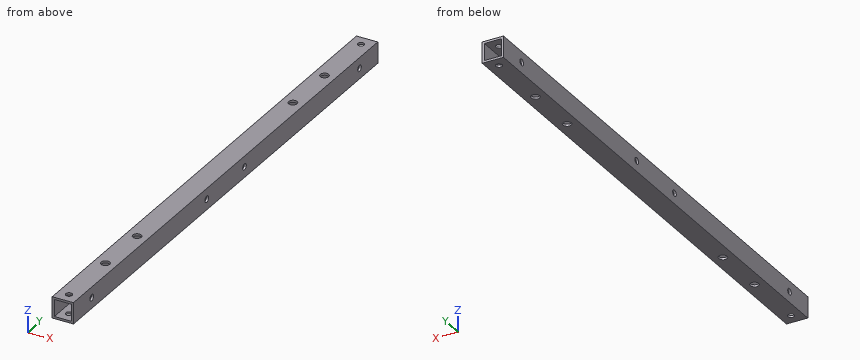
```python
from build123d import *

# Parameters (mm, degrees)
F0_W     = 10
F0_H     = 10
F0_W_2   = 8
F0_H_2   = 8
F1_DEPTH = 250
F2_R     = 1.5
F4_DEPTH = 25
F3_R     = 1.5
F3_R_2   = 2
F5_DEPTH = 25


with BuildPart() as f1:
    # F0 (on Front) → F1 (new body)
    with BuildSketch(Plane.XZ):
        Rectangle(F0_W, F0_H)
        Rectangle(F0_W_2, F0_H_2, mode=Mode.SUBTRACT)
    extrude(amount=F1_DEPTH)

    # F2 (on face) → F4 (cut)
    with BuildSketch(Plane.YZ.offset(5)):
        with Locations((-140.5, 0)):
            Circle(F2_R)
        with Locations((-235, 0)):
            Circle(F2_R)
        with Locations((-15, 0)):
            Circle(F2_R)
        with Locations((-109.5, 0)):
            Circle(F2_R)
    extrude(amount=-F4_DEPTH, mode=Mode.SUBTRACT)

    # F3 (on face) → F5 (cut)
    with BuildSketch(Plane.XY.offset(5)):
        with Locations((0, -245)):
            Circle(F3_R)
        with Locations((0, -215)):
            Circle(F3_R_2)
        with Locations((0, -189)):
            Circle(F3_R_2)
        with Locations((0, -61)):
            Circle(F3_R_2)
        with Locations((0, -35)):
            Circle(F3_R_2)
        with Locations((0, -5)):
            Circle(F3_R)
    extrude(amount=-F5_DEPTH, mode=Mode.SUBTRACT)


solid = f1.part
```
Geometry: final body of the model. Coordinates: model frame, mm. Coordinates: 2 decimals unless noted, no trailing zeros. Order: outer loops, then holes, each group sorted by start corner. A loop starts at its lowest first (then second) coordinate and runs counter-clockwise, first axis right, second up. Notation, with made-up numbers: (-32.75, -29.75) - (-11.75, -29.75) arc R22 ccw to (-11.75, -19.75) - close; hole circle Ø9 at (86, 36.25). An arc over 180 degrees is marked (long way). Return JSON: item names as keys, results as strings. Group by question number.
1. Pin query (flat end, axial travel): pin 1 (2.5 mm diameter, centred on y = -109.5, z = 0, fed in from +X). Return the tip coordinate at first contact, or that it passes through.
2. Cut plane A-A (y = -170). Output: boundary loops of the cut face in (x, z).
3. Material intervals for line 1 along X through (y, z) = (-199.5, 3.75); line 2 along X through (y, z) = (-215, 4.8), sorted ascending. Write a range as [from, to].
4. Cut plane B-B (z = 0). Count the separate pieces of the cut face and the enclosed holes in it, plus the area to 3 significant figures.
Resolved:
{
 "1": {"pin 1": "passes through"},
 "2": {"outline": "(-5, -5) - (5, -5) - (5, 5) - (-5, 5) - close; hole (-4, -4) - (4, -4) - (4, 4) - (-4, 4) - close"},
 "3": {"line 1": "x = [-5, -4], [4, 5]", "line 2": "x = [-5, -2], [2, 5]"},
 "4": {"separate pieces": "10", "enclosed holes": "0", "area": "476 mm²"}
}
